The listing builds one solid part. Answer for the finished solid, in the listing's coordinates (mm). Face numbers are marked on the shaded views. Round coordinates to 2 decimals unless told otherwise and drop trailing zeros. Order: outer loops, then holes, each group sorted by start corner. A loop starts at its lowest first (then second) coordinate and runs counter-clockwise, first axis right, second up. Notation, with made-up numbers: (69, 49.25) -> (116, 49.25) arc R26 ccw to (116, 69.25) -> close; hole circle Ø4 at (-19, 16.25). An arc over 180 degrees is marked (long way). Return JSON: item names as keys, results as strings. Group by question number.
(1) The part is cut by section A-A (z = 3.5). Count the separate pieces of the cut face and the enclosed holes in it, plus the area to 3 significant figures.
(2) The part is cut by section B-B (y = 18.5). Determine the outline of the cut face in (x, z).
(3) The part is cut by section D-D (y = -13.5). Determine the outline of the cut face in (x, z), plus the area to 3 significant figures.
(4) Each of these flat-tipped pins is pushed along its axis until it touches: pin 1 (6 mm diameter, centred on x = -31.5, z = 4.5, fed in from -Y); pin 2 (10 mm diameter, centred on x = -16.5, z = 8, fed in from -Y); pin 3 (5 mm diameter, centred on x = -25, z = 11, fed in from -Y). Where does it stop, or does it pass through?
(5) Consider line 1 (X direction, y = -26, z = 13); line 2 (X direction, y = 19, z = 9); line 3 (Y direction, x = 23, z = 12.5). Determine where each line is inside the solid, lowest interval first. Write a range as [from, to].
(6) Determine the mould class of the marked faces 1 and 2 for opening direction Y: +Y half, -Y half, draft (parallel to the pull), parting line (faces both ways), or undercut.
(7) The part is cut by section C-C (y = -33). Determine the outline of the cut face in (x, z).
Autodesk Inventor part; units mm, degrees
ref_plane "YZ Plane" through (0, 0, 0) normal (1, 0, 0) x (0, 1, 0)
ref_plane "XZ Plane" through (0, 0, 0) normal (0, 1, 0) x (-1, 0, 0)
ref_plane "XY Plane" through (0, 0, 0) normal (0, 0, 1) x (1, 0, 0)
sketch "Sketch1" plane through (0, 0, 0) normal (0, 0, 1) x (1, 0, 0)
  line L0 (0, 66.675) -> (0, -66.675)
  line L1 (-66.675, 0) -> (66.675, 0)
  circle A0 centre (0, 0) radius 47.625
  circle A1 centre (0, 0) radius 10.3188
  dimension "d0" = 20.6375
  dimension "d1" = 95.25
extrude "Extrusion1" add sketch "Sketch1" along normal blind 20.574
sketch "Sketch2" plane through (0, 0, 0) normal (0, 0, -1) x (-1, 0, 0)
  line L0 (0, -66.675) -> (0, 66.675)
  line L1 (-66.675, 0) -> (66.675, 0)
  line L2 (-24.1554, -24.1554) -> (24.1554, -24.1554) construction
  line L3 (24.1554, -24.1554) -> (24.1554, 24.1554) construction
  line L4 (24.1554, 24.1554) -> (-24.1554, 24.1554) construction
  line L5 (-24.1554, 24.1554) -> (-24.1554, -24.1554) construction
  line L6 (-24.1554, -24.1554) -> (24.1554, 24.1554) construction
  line L7 (24.1554, -24.1554) -> (-24.1554, 24.1554) construction
  circle A0 centre (0, 0) radius 34.1609 construction
  dimension "d25" = 68.3218
  dimension "d22" = 48.3108
hole "Hole1" at (-24.1554, -24.1554, 0) direction (0, 0, 1) diameter 4.134 end through all
sketch "Sketch3" plane through (0, 0, 20.574) normal (0, 0, 1) x (1, 0, 0)
  line L0 (0, 66.675) -> (0, -66.675)
  line L1 (-66.675, 0) -> (66.675, 0)
  circle A0 centre (0, 0) radius 41.275 construction
  line L2 (0, 0) -> (-36.6114, -19.0587) construction
  point P0 (-24.1554, -24.1554)
  point P1 (-24.1554, -24.1554)
  dimension "d23" = 82.55
  dimension "d24" = 62.5
hole "Hole2" at (-36.6114, -19.0587, 20.574) direction (0, 0, -1) diameter 4.917 end through all
pattern_circular "Circular Pattern1" count 4 over 360 about axis through (0, 0, -10) along (0, 0, 1) of "Hole1", "Hole2"
properties part number "J010343" material "ALUMINUM, 6061-T651"
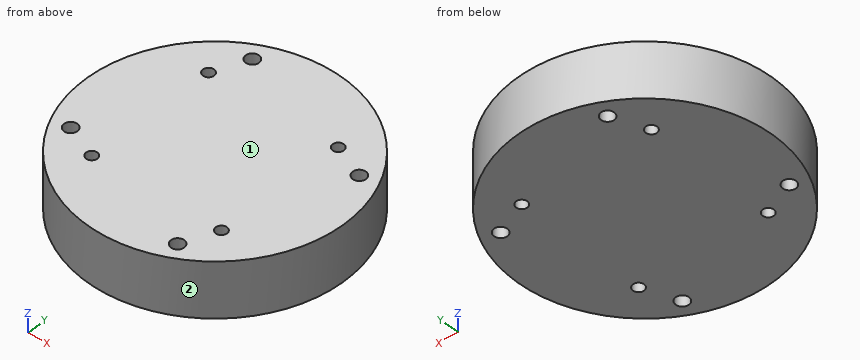
Answer below:
{
 "1": {"separate pieces": "1", "enclosed holes": "8", "area": "7,000 mm²"},
 "2": {"outline": "(-43.88, 0) -> (34.22, 0) -> (34.22, 20.57) -> (-43.88, 20.57) -> close; (39.01, 0) -> (43.88, 0) -> (43.88, 20.57) -> (39.01, 20.57) -> close"},
 "3": {"outline": "(-45.67, 0) -> (45.67, 0) -> (45.67, 20.57) -> (-45.67, 20.57) -> close", "area": "1,880 mm²"},
 "4": {"pin 1": "stops at y = -38.16", "pin 2": "stops at y = -46.22", "pin 3": "stops at y = -41.97"},
 "5": {"line 1": "x = [-39.9, -25.09], [-23.22, 23.22], [25.09, 39.9]", "line 2": "x = [-43.67, 34.15], [39.07, 43.67]", "line 3": "y = [-41.7, -25.87], [-22.44, 22.44], [25.87, 41.7]"},
 "6": {"face 1": "draft", "face 2": "parting line"},
 "7": {"outline": "(-34.34, 0) -> (34.34, 0) -> (34.34, 20.57) -> (-34.34, 20.57) -> close"}
}
